```python
from build123d import *

# Parameters (mm, degrees)
F0_R      = 56.323748
F1_DEPTH  = 2
F2_R      = 36.666383
F3_DEPTH  = 2
F4_R      = 25.730938
F5_DEPTH  = 2
F6_R      = 12.6095
F7_DEPTH  = 2
F8_R      = 7.082523
F9_DEPTH  = 2
F10_R     = 4.140126
F11_DEPTH = 3


with BuildPart() as f1:
    # F0 (on Top) → F1 (new body)
    with BuildSketch(Plane.XY):
        Circle(F0_R)
    extrude(amount=F1_DEPTH)

    # F2 (on face) → F3 (join)
    with BuildSketch(Plane.XY.offset(2)):
        Circle(F2_R)
    extrude(amount=F3_DEPTH)

    # F4 (on face) → F5 (join)
    with BuildSketch(Plane.XY.offset(4)):
        Circle(F4_R)
    extrude(amount=F5_DEPTH)

    # F6 (on face) → F7 (join)
    with BuildSketch(Plane.XY.offset(6)):
        with Locations((3.81, 4.884616)):
            Circle(F6_R)
    extrude(amount=F7_DEPTH)

    # F8 (on face) → F9 (join)
    with BuildSketch(Plane.XY.offset(8)):
        with Locations((3.81, 4.884616)):
            Circle(F8_R)
    extrude(amount=F9_DEPTH)

    # F10 (on face) → F11 (join)
    with BuildSketch(Plane.XY.offset(10)):
        with Locations((3.81, 4.884616)):
            Circle(F10_R)
    extrude(amount=F11_DEPTH)


solid = f1.part
```
Verification items for the finished model (mm, model axes). A direction names the side the tool comes from. Coordinates: 2 decimals unless noted, no trailing zeros. Loops run counter-clockwise (first coordinate to the right, second up) from the corner with the lowest first, then second, coordinate; pieces in that order, holes last. Notation, with made-up numbers: (-34, 45.25) -> (21, 45.25) arc R22 ccw to (21, 62.25) -> close; hole circle Ø11 at (49.5, 61.5). An arc over 180 degrees is marked (long way). Answer in a Markdown table with one row per item. Add a question column.
1. Section check D-D, the plane y = 33. Enter the section's corners in (x, z).
2. Material ranges on probe 1 along Z at (x, y) = (-46, 31); probe 2 along Z at (x, y) = (23.5, -20); probe 3 along Y at (x, z) = (12, 4.5), recorded low to high. Write a range as [from, to].
3. Access from +Z, -Z, +X, -X, +Y, -Y to the whole of each face (thin tool, end or side, straight path). Record for faces 1 (the face through (8, 25, 4)), 2 (the face through (-1, 1, 0)).
4. Section check B-B, the plane y = 19. Enter the section's corners in (x, z).
5. Depth check by flat-ended pin: P1, Ø20, axis at x = 6.5, y = 10.5, coming from the +Z side; P2, Ø5, axis at x = -21.5, z = 5, coming from the -Y side; P3, Ø1, axis at x = 26, y = 2.5, coming from the +Z side; P4, Ø6, axis at x = 33, z = 9, coming from the -Y side (3 decimals). Enter the tip coordinate at first touch or a pass-through.
6. Section check C-C, the plane x = 35. Enter the section's corners in (y, z).
7. Section check A-A, the plane x = 3. Enter the section's corners in (y, z).
Derived:
| question | item | result |
|---|---|---|
| 1 | outline | (-45.64, 0) -> (45.64, 0) -> (45.64, 2) -> (15.98, 2) -> (15.98, 4) -> (-15.98, 4) -> (-15.98, 2) -> (-45.64, 2) -> close |
| 2 | probe 1 | z = [0, 2] |
| 2 | probe 2 | z = [0, 4] |
| 2 | probe 3 | y = [-22.76, 22.76] |
| 3 | face 1 | +Z |
| 3 | face 2 | -Z, +X, -X, +Y, -Y |
| 4 | outline | (-53.02, 0) -> (53.02, 0) -> (53.02, 2) -> (31.36, 2) -> (31.36, 4) -> (17.35, 4) -> (17.35, 6) -> (-17.35, 6) -> (-17.35, 4) -> (-31.36, 4) -> (-31.36, 2) -> (-53.02, 2) -> close |
| 5 | P1 | stops at z = 13 |
| 5 | P2 | stops at y = -31.23 |
| 5 | P3 | stops at z = 6 |
| 5 | P4 | passes through |
| 6 | outline | (-44.13, 0) -> (44.13, 0) -> (44.13, 2) -> (10.93, 2) -> (10.93, 4) -> (-10.93, 4) -> (-10.93, 2) -> (-44.13, 2) -> close |
| 7 | outline | (-56.24, 0) -> (56.24, 0) -> (56.24, 2) -> (36.54, 2) -> (36.54, 4) -> (25.56, 4) -> (25.56, 6) -> (17.47, 6) -> (17.47, 8) -> (11.92, 8) -> (11.92, 10) -> (8.94, 10) -> (8.94, 13) -> (0.82, 13) -> (0.82, 10) -> (-2.15, 10) -> (-2.15, 8) -> (-7.7, 8) -> (-7.7, 6) -> (-25.56, 6) -> (-25.56, 4) -> (-36.54, 4) -> (-36.54, 2) -> (-56.24, 2) -> close |
